from build123d import *

# Parameters (mm, degrees)
SKETCH_1_W      = 28
SKETCH_1_H      = 28
SKETCH_1_W_2    = 18
SKETCH_1_H_2    = 25.4
SKETCH_1_W_3    = 7.4
EXTRUDE_1_DEPTH = 1
SKETCH_1_3_W    = 25.4
SKETCH_1_3_H    = 25.4
EXTRUDE_2_DEPTH = 4
SKETCH_1_4_W    = 18.5
SKETCH_1_4_H    = 26
EXTRUDE_3_DEPTH = 4
FILLET_1_R      = 3


with BuildPart() as part:
    # Sketch 1 → Extrude 1 (new body)
    # profile 1 of 4: a face of its own
    with BuildSketch(Plane(origin=(0, 0, 0), x_dir=(1, 0, 0), z_dir=(0, 1, 0))):
        Rectangle(SKETCH_1_W, SKETCH_1_H)
        Polygon((6, 13), (6, 12.7), (13.4, 12.7), (13.4, -12.7), (6, -12.7), (6, -13), (-12.5, -13), (-12.5, 13), align=None, mode=Mode.SUBTRACT)
    # profile 2 of 4: a face of its own
    with BuildSketch(Plane(origin=(0, 0, 0), x_dir=(1, 0, 0), z_dir=(0, 1, 0))):
        with Locations((-3, 0)):
            Rectangle(SKETCH_1_W_2, SKETCH_1_H_2)
    # profile 3 of 4: a face of its own
    with BuildSketch(Plane(origin=(0, 0, 0), x_dir=(1, 0, 0), z_dir=(0, 1, 0))):
        Polygon((-12, -12.7), (-12, 12.7), (6, 12.7), (6, 13), (-12.5, 13), (-12.5, -13), (6, -13), (6, -12.7), align=None)
    # profile 4 of 4: a face of its own
    with BuildSketch(Plane(origin=(0, 0, 0), x_dir=(1, 0, 0), z_dir=(0, 1, 0))):
        with Locations((9.7, 0)):
            Rectangle(SKETCH_1_W_3, SKETCH_1_H_2)
    extrude(amount=EXTRUDE_1_DEPTH)

    # Sketch 1_3 → Extrude 2 (add)
    with BuildSketch(Plane(origin=(0, 0, 0), x_dir=(1, 0, 0), z_dir=(0, 1, 0))):
        with Locations((0.7, 0)):
            Rectangle(SKETCH_1_3_W, SKETCH_1_3_H)
    extrude(amount=-EXTRUDE_2_DEPTH)

    # Sketch 1_4 → Extrude 3 (add)
    with BuildSketch(Plane(origin=(0, 0, 0), x_dir=(1, 0, 0), z_dir=(0, 1, 0))):
        with Locations((-3.25, 0)):
            Rectangle(SKETCH_1_4_W, SKETCH_1_4_H)
    extrude(amount=EXTRUDE_3_DEPTH)

    # Fillet 1
    fillet_1_edges = [part.edges().sort_by_distance(p)[0] for p in [
        (-12, -2, -12.7),
        (13.4, -2, -12.7),
        (13.4, -2, 12.7),
        (-12, -2, 12.7),
    ]]
    fillet(fillet_1_edges, radius=FILLET_1_R)


solid = part.part
CAD build for the part. Positions are in the model's coordinates, mm. A direction names the side the tool comes from. Round coordinates to 2 decimals unless told otherwise and drop trailing zeros. Write each loop counter-clockwise with the first axis right and the second up, starting at its lowest first coordinate (ties: lowest second). Pieces come first, ordered by that corner, then holes.
(1) 3-axis set-ups, long thin cutter, end or side, ignore diameter. For faces 1 (the face through (-3, 2, -13)), 2 (the face through (-12.5, 2, 0)), 3 (the face through (-13, 0, 1)), 4 (the face through (-11.14, -2.03, 11.8)): which of +Z, -Z, +X, -X, +Y, -Y reach the whole face in a straight line?
(2) Slice it at C-C, the plane z = -3. Write the cut outline in (x, y).
(3) Slice it at B-B, the plane y = -2.5. Write the cut outline in (x, z).
(4) Drop flat-ended pins along their axis: P1, Ø0.9, axis at y = 2.5, z = 1.5, coming from the +X side; P2, Ø3, axis at y = -2, z = 4, coming from the -X side; P3, Ø0.9, axis at y = 2.5, z = 2, coming from the -X side. Give the stop position or say it passes through.
(5) Probe line 1 along Z through (x, y) = (4.5, 2.75); line 2 along X through (y, z) = (-3, -3.75); line 3 along X through (y, z) = (3.5, 2.5). List the from-to ranges inside material, lowest first.
(6) Slice it at D-D, the plane x = 11.25. Write the cut outline in (y, z), and give its area (3 significant figures).
(7) Slice it at A-A, the plane x = -5.5. Write the cut outline in (y, z).
From the geometry:
1. face 1: -Z, +X, -X, +Y
1. face 2: +Z, -Z, -X, +Y
1. face 3: -Y
1. face 4: +Z, -X, -Y
2. outline: (-14, 0) - (-12, 0) - (-12, -4) - (13.4, -4) - (13.4, 0) - (14, 0) - (14, 1) - (6, 1) - (6, 4) - (-12.5, 4) - (-12.5, 1) - (-14, 1) - close
3. outline: (-12, -9.7) arc R3 ccw to (-9, -12.7) - (10.4, -12.7) arc R3 ccw to (13.4, -9.7) - (13.4, 9.7) arc R3 ccw to (10.4, 12.7) - (-9, 12.7) arc R3 ccw to (-12, 9.7) - close
4. P1: stops at x = 6
4. P2: stops at x = -12
4. P3: stops at x = -12.5
5. line 1: z = -13 to 13
5. line 2: x = -12 to 13.4
5. line 3: x = -12.5 to 6
6. outline: (-4, -12.58) - (0, -12.58) - (0, -14) - (1, -14) - (1, 14) - (0, 14) - (0, 12.58) - (-4, 12.58) - close
6. area: 129 mm2
7. outline: (-4, -12.7) - (0, -12.7) - (0, -14) - (1, -14) - (1, -13) - (4, -13) - (4, 13) - (1, 13) - (1, 14) - (0, 14) - (0, 12.7) - (-4, 12.7) - close
